Build history of the part. All positions in model axes, mm. A direction names the side the tool comes from. Give positions to 0.01 mm unless a question says otherwise; leave off trailing zeros. Write each loop counter-clockwise with the first axis right and the second up, starting at its lowest first coordinate (ties: lowest second). Pieces come first, ordered by that corner, then holes. Notation, with made-up numbers: M -7,40.5 L 46,40.5 A5 ccw 46,45.5 Z; hole C -15,80.25 d11. An arc over 180 degrees is marked long. Return JSON: item names as keys, results as strings. Group by question number.
Q1. Wall check: probe 1 along X at (y, z) = (-8.89, 2.85); probe 2 along Z at (x, y) = (-2.25, 0.75); probe 3 along Z at (x, y) = (-1.5, -1). Give the ranges that are in metal, low to high.
Q2. Pull direction X, two halves, no side cores. Call faces 1 (the cylindrical face through (2.224, -8.966, 3.352)), 2 (the cylindrical face through (0.13, -5.81, 6.35)), 3 (the flat face through (0, -7, 0.635)): +X half, -X half, draft (parallel to the pull), parting line (faces both ways), or undercut.
Q3. Band-saw the part on B-B, the plane x = -3. Give the cut face in (y, z) (3 decimals), then the cut area to 3 significant figures.
Q4. Band-saw the part on D-D, the plane z = 3.7. Give the cut face in (x, y).
Q5. Band-saw the part on A-A, the plane y = -8.89. Count the separate pieces of the cut face and the enclosed holes in it, then the cut area to 3 significant figures.
Q6. Tool access for faces 4 (the flat face through (3, -9, 1.651)), 5 (the flat face through (0, -12.7, 3)): list every direction of +Z, -Z, +X, -X, +Y, -Y with a clear straight run to the whole face (end or side of a thin tool).
Q7. Flat gauge pins, fed straight in: pin 1 Ø5 at (x, y) = (4, -4.5) entering from +Z; pin 2 Ø3 at (x, y) = (-4.64, -8.89) entering from +Z; pin 3 Ø3.5 at (x, y) = (-4.64, -8.89) entering from -Z (3 decimals); pin 4 Ø1.5 at (y, z) = (-2, 2) entering from -X. Where does each tip first touch, or does it go through?
Q8. Band-saw the part on C-C, the plane z = 1.2. Give the cut face in (x, y), then the cut area to 3 significant figures.
from build123d import *

# Parameters (mm, degrees)
BOSS_EXTRUDE1_DEPTH = 13.97
FILLET1_R           = 2.54
SKETCH4_R           = 1.4732
CUT_EXTRUDE1_DEPTH  = 6.7150001
SKETCH6_R           = 2.413
CUT_EXTRUDE3_DEPTH  = 5.334


with BuildPart() as part:
    # Sketch3 → Boss-Extrude1 (new body)
    with BuildSketch(Plane.XZ.offset(12.7)):
        with BuildLine():
            ThreePointArc((6.318170226, 0.635), (0, 6.35), (-6.318170226, 0.635))
            Line((-6.318170226, 0.635), (6.318170226, 0.635))
        make_face()
    extrude(amount=-BOSS_EXTRUDE1_DEPTH)

    # Fillet1
    fillet1_edges = [part.edges().sort_by_distance(p)[0] for p in [
        (0, 1.27, 0.635),
    ]]
    fillet(fillet1_edges, radius=FILLET1_R)

    # Sketch4 → Cut-Extrude1 (cut, through all)
    with BuildSketch(Plane(origin=(0, 0, 0.635), x_dir=(-1, 0, 0), z_dir=(0, 0, -1))):
        with Locations((4.6355, -8.89)):
            Circle(SKETCH4_R)
        with Locations((-4.6355, -8.89)):
            Circle(SKETCH4_R)
    extrude(amount=-CUT_EXTRUDE1_DEPTH, mode=Mode.SUBTRACT)

    # Sketch6 → Cut-Extrude3 (cut)
    with BuildSketch(Plane(origin=(0, 0, 6.985), x_dir=(-1, 0, 0), z_dir=(0, 0, -1))):
        with Locations((4.6355, -8.89)):
            Circle(SKETCH6_R)
        with Locations((-4.6355, -8.89)):
            Circle(SKETCH6_R)
    extrude(amount=CUT_EXTRUDE3_DEPTH, mode=Mode.SUBTRACT)


solid = part.part
From the geometry:
{
 "1": {"probe 1": "x = -2.22 to 2.22", "probe 2": "z = 1.64 to 5.94", "probe 3": "z = 0.65 to 6.17"},
 "2": {"face 1": "undercut", "face 2": "parting line", "face 3": "draft"},
 "3": {"outline": "M -12.7,0.635 L -1.27,0.635 A2.54 ccw 1.27,3.175 L 1.27,5.597 L -7.116,5.597 L -7.116,1.651 L -10.664,1.651 L -10.664,5.597 L -12.7,5.597 Z", "area": "53.9 mm^2"},
 "4": {"outline": "M -5.16,-12.7 L 5.16,-12.7 L 5.16,-11.25 A2.41 cw long 5.16,-6.53 L 5.16,1.27 L -5.16,1.27 L -5.16,-6.53 A2.41 cw long -5.16,-11.25 Z"},
 "5": {"separate pieces": "3", "enclosed holes": "0", "area": "27.0 mm^2"},
 "6": {"face 4": "+Z", "face 5": "+Z, -Z, +X, -X, -Y"},
 "7": {"pin 1": "stops at z = 6.17", "pin 2": "stops at z = 1.65", "pin 3": "stops at z = 0.635", "pin 4": "stops at x = -6.23"},
 "8": {"outline": "M -6.24,-12.7 L 6.24,-12.7 L 6.24,0.33 L -6.24,0.33 Z; hole C -4.64,-8.89 d2.95; hole C 4.64,-8.89 d2.95", "area": "149 mm^2"}
}
